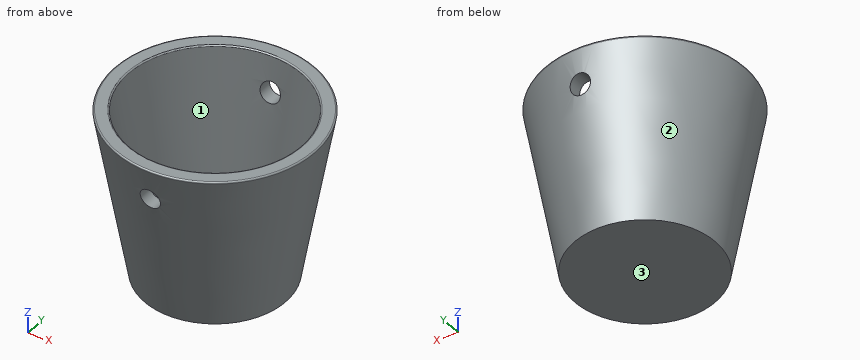
```python
from build123d import *

# Parameters (mm, degrees)
F2_T     = -5.08
F3_R     = 3.81
F4_DEPTH = 254
F5_DEPTH = 254
F6_R     = 0.508


with BuildPart() as f1:
    # F0 (on Front) → F1 (revolve)
    with BuildSketch(Plane.XZ):
        Polygon((0, 0), (0, 63.5), (-38.1, 63.5), (-26.903236725, 0), align=None)
    revolve(axis=Axis((0, 0, 31.75), (0, 0, 1)))

    # F2
    f2_openings = [f1.faces().sort_by_distance(p)[0] for p in [
        (0, 0, 63.5),
    ]]
    offset(amount=F2_T, openings=f2_openings)

    # F3 (on Front) → F4 (cut)
    with BuildSketch(Plane.XZ):
        with Locations((0, 50.8)):
            Circle(F3_R)
    extrude(amount=-F4_DEPTH, mode=Mode.SUBTRACT)

    # F3 (on Front) → F5 (cut)
    with BuildSketch(Plane.XZ):
        with Locations((0, 50.8)):
            Circle(F3_R)
    extrude(amount=F5_DEPTH, mode=Mode.SUBTRACT)

    # F6
    f6_edges = [f1.edges().sort_by_distance(p)[0] for p in [
        (38.1, 0, 63.5),
        (32.941633, 0, 63.5),
    ]]
    fillet(f6_edges, radius=F6_R)


solid = f1.part
```
Model file for the job. Use its own axes, mm. Face numbers are marked on the shaded views. Round coordinates to 2 decimals unless told otherwise and drop trailing zeros. Loops run counter-clockwise (first coordinate to the right, second up) from the corner with the lowest first, then second, coordinate; pieces in that order, holes last. Notation, with made-up numbers: M 9.5,74 L 29.5,74 A13 cw 29.5,87 Z; hole C 17,-14 d2. An arc over 180 degrees is marked long. Put each result on its own line as item: value. Start each with the question number.
Item 1: Mould opens along X. For the marked faces 1, 2 and 3 say: released by +X, released by -X, zero draft, split by the parting line, or undercut.
Item 2: Drop flat-ended pins along their axis: P1, Ø3, axis at y = 30, z = 34, coming from the +X side; P2, Ø8, axis at x = 30, y = 13.5, coming from the +Z side; P3, Ø8, axis at x = -26, z = 42.5, coming from the +Y side; P4, Ø12, axis at x = 0, z = 50.8, coming from the +Y side. Give the stop position or say it passes through.
Item 3: Cut at A-A (x = 0). List the corners of the cut face in (y, z), then the cut area to 3 significant figures.
Item 4: Drill centre lines: line 1 along X through (y, z) = (-18, 20.5); line 2 along X through (y, z) = (7.5, 17); line 3 along Y through (x, z) = (-19, 11.5). Where is each one in solid material? Low to high.
Item 5: Cut at D-D (z = 29). List the corners of the cut face in (x, y), then the cut area to 3 significant figures.
Item 6: Cut at C-C (y = 0). List the corners of the cut face in (x, z).
Answer block:
1. face 1: undercut
1. face 2: split by the parting line
1. face 3: zero draft
2. P1: x = 16.49
2. P2: z = 63.5
2. P3: y = 26.57
2. P4: y = 36.92
3. outline: M -37.99,62.9 L -36.53,54.61 L -31.37,54.61 L -32.87,63.08 A0.51 ccw -33.37,63.5 L -37.49,63.5 A0.51 ccw Z; M -35.19,46.99 L -26.9,0 L 26.9,0 L 35.19,46.99 L 30.03,46.99 L 22.64,5.08 L -22.64,5.08 L -30.03,46.99 Z; M 31.37,54.61 L 36.53,54.61 L 37.99,62.9 A0.51 ccw 37.49,63.5 L 33.37,63.5 A0.51 ccw 32.87,63.08 Z
3. area: 802 mm2
4. line 1: -24.64 to -17.86, 17.86 to 24.64
4. line 2: -28.94 to -23.58, 23.58 to 28.94
4. line 3: -21.82 to -14.29, 14.29 to 21.82
5. outline: C 0,0 d64.03; hole C 0,0 d53.72
5. area: 954 mm2
6. outline: M -37.99,62.9 L -26.9,0 L 26.9,0 L 37.99,62.9 A0.51 ccw 37.49,63.5 L 33.37,63.5 A0.51 ccw 32.87,63.08 L 22.64,5.08 L -22.64,5.08 L -32.87,63.08 A0.51 ccw -33.37,63.5 L -37.49,63.5 A0.51 ccw Z
